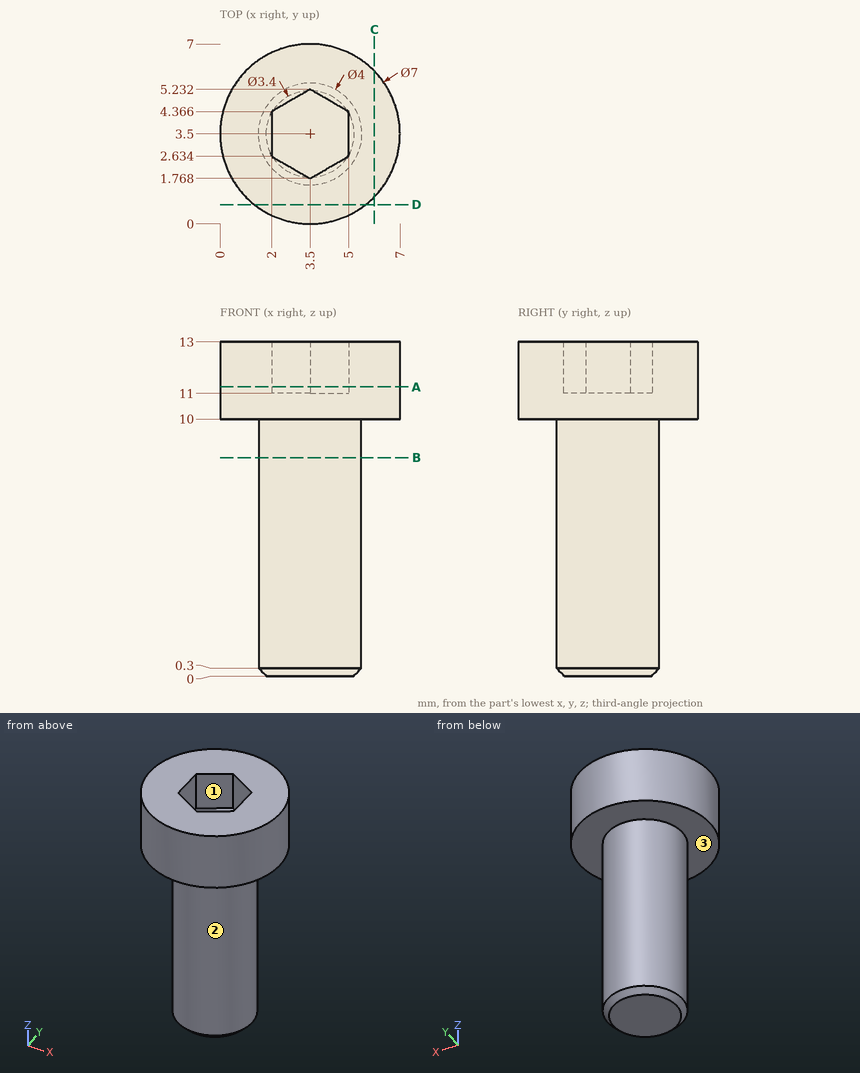
Answer from the drawing. Dimensions are ordinates in mm from the lowest x, y and z of the part. Round coordinates to 2 decimals unless told otherwise and drop trailing zeros. Write each loop counter-clockwise with the first axis right and the second up, starting at its lowest first coordinate (ties: lowest second). Pieces come first, ordered by that corner, then holes.
1. Given pin 1 Ø1.5 at (y, z) = (2, 8) entering from -X; pin 2 Ø4 at (y, z) = (2, 8.5) entering from +X, each flat-ended and moving along its own axis, determine where each tip first touches the part or whether it passes through.
2. The part is cut by section A-A, the plane z = 11.25. Determine the outline of the cut face in (x, y).
3. The part is cut by section C-C, the plane x = 6. Determine the outline of the cut face in (y, z), then the cut area to 3 significant figures.
4. Straight lines are drawn through the part: L1, parallel to Y at x = 2.5, z = 2; L2, parallel to Z at x = 4.5, y = 1.25. For each, find the intervals that lie inside material, in ascending order.
5. Determine the mould class of the marked faces 1, 2 and 3 for opening direction X: pulls with the +X half, pulls with the -X half, needs draft (parallel to the pull), parting line crosses it, or undercut.
6. The part is cut by section B-B, the plane z = 8.5. Determine the outline of the cut face in (x, y), then the cut area to 3 significant figures.
7. The part is cut by section D-D, the plane y = 0.75. Determine the outline of the cut face in (x, z) (3 decimals).
Values:
1. pin 1: stops at x = 1.65
1. pin 2: stops at x = 7
2. outline: circle Ø7 at (3.5, 3.5); hole (2, 2.63) - (3.5, 1.77) - (5, 2.63) - (5, 4.37) - (3.5, 5.23) - (2, 4.37) - close
3. outline: (1.05, 10) - (5.95, 10) - (5.95, 13) - (1.05, 13) - close
3. area: 14.7 mm2
4. L1: y = 1.77 to 5.23
4. L2: z = 10 to 13
5. face 1: undercut
5. face 2: parting line crosses it
5. face 3: needs draft
6. outline: circle Ø4 at (3.5, 3.5)
6. area: 12.6 mm2
7. outline: (1.335, 10) - (5.665, 10) - (5.665, 13) - (1.335, 13) - close
